```python
from build123d import *

# Parameters (mm, degrees)
SKETCH_1_W           = 150
SKETCH_1_H           = 150
EXTRUDE_2_DEPTH      = 55
CUT_EXTRUDE_1_DEPTH  = 52
SKETCH_3_W           = 20
SKETCH_3_H           = 25.2
CUT_EXTRUDE_2_DEPTH  = 52
SKETCH_4_W           = 31.2
SKETCH_4_H           = 23.663491794
CUT_EXTRUDE_3_DEPTH  = 52
SKETCH_5_W           = 46
SKETCH_5_H           = 120
SKETCH_5_W_2         = 29
CUT_EXTRUDE_4_DEPTH  = 40
SKETCH_6_W           = 3
SKETCH_6_H           = 120
EXTRUDE_4_DEPTH      = 25
SKETCH_7_W           = 3
SKETCH_7_H           = 120
EXTRUDE_5_DEPTH      = 20
CUT_EXTRUDE_6_DEPTH  = 30
FILLET_1_R           = 7
SKETCH_10_W          = 80
SKETCH_10_H          = 50
CUT_EXTRUDE_7_DEPTH  = 30
SKETCH_11_W          = 11.4
SKETCH_11_H          = 20
CUT_EXTRUDE_8_DEPTH  = 30
FILLET_2_R           = 5
FILLET_3_R           = 2
SKETCH_12_W          = 12.6
SKETCH_12_H          = 20
CUT_EXTRUDE_9_DEPTH  = 20
FILLET_4_R           = 2
SKETCH_13_R          = 0.75
CUT_EXTRUDE_10_DEPTH = 5
FILLET_5_R           = 2
FILLET_6_R           = 1
FILLET_8_R           = 0.3


with BuildPart() as part:
    # 草图1 → 凸台-拉伸2 (new body)
    with BuildSketch(Plane.XY):
        with Locations((75, -75)):
            Rectangle(SKETCH_1_W, SKETCH_1_H)
    extrude(amount=EXTRUDE_2_DEPTH)

    # 草图2 → 切除-拉伸1 (cut)
    with BuildSketch(Plane(origin=(0, 0, 0), x_dir=(-1, 0, 0), z_dir=(0, 0, -1))):
        Polygon((-57.4, -53), (-92.6, -53), (-97, -57.4), (-97, -92.6), (-92.6, -97), (-57.4, -97), (-53, -92.6), (-53, -57.4), align=None)
    extrude(amount=-CUT_EXTRUDE_1_DEPTH, mode=Mode.SUBTRACT)

    # 草图3 → 切除-拉伸2 (cut)
    with BuildSketch(Plane(origin=(0, 0, 0), x_dir=(-1, 0, 0), z_dir=(0, 0, -1))):
        with Locations((-43, -75)):
            Rectangle(SKETCH_3_W, SKETCH_3_H)
    extrude(amount=-CUT_EXTRUDE_2_DEPTH, mode=Mode.SUBTRACT)

    # 草图4 → 切除-拉伸3 (cut)
    with BuildSketch(Plane(origin=(0, 0, 0), x_dir=(-1, 0, 0), z_dir=(0, 0, -1))):
        with Locations((-75, -41.168254103)):
            Rectangle(SKETCH_4_W, SKETCH_4_H)
    extrude(amount=-CUT_EXTRUDE_3_DEPTH, mode=Mode.SUBTRACT)

    # 草图5 → 切除-拉伸4 (cut)
    with BuildSketch(Plane(origin=(0, 0, 0), x_dir=(-1, 0, 0), z_dir=(0, 0, -1))):
        with Locations((-127, -75)):
            Rectangle(SKETCH_5_W, SKETCH_5_H)
        with Locations((-164.5, -75)):
            Rectangle(SKETCH_5_W_2, SKETCH_5_H)
    extrude(amount=-CUT_EXTRUDE_4_DEPTH, mode=Mode.SUBTRACT)

    # 草图6 → 凸台-拉伸4 (add)
    with BuildSketch(Plane(origin=(150, 0, 0), x_dir=(0, 0, -1), z_dir=(1, 0, 0))):
        Polygon((-43, -15), (-40, -15), (0, -15), (0, -12), (-43, -12), align=None)
        with Locations((-41.5, -75)):
            Rectangle(SKETCH_6_W, SKETCH_6_H)
        Polygon((0, -135), (-40, -135), (-43, -135), (-43, -138), (0, -138), align=None)
    extrude(amount=EXTRUDE_4_DEPTH)

    # 草图7 → 凸台-拉伸5 (add)
    with BuildSketch(Plane(origin=(0, 0, 40), x_dir=(-1, 0, 0), z_dir=(0, 0, -1))):
        with Locations((-173.5, -75)):
            Rectangle(SKETCH_7_W, SKETCH_7_H)
    extrude(amount=EXTRUDE_5_DEPTH)

    # 草图8 → 切除-拉伸6 (cut)
    with BuildSketch(Plane(origin=(0, 0, 0), x_dir=(-1, 0, 0), z_dir=(0, 0, -1))):
        Polygon((-69, -15), (-104, -15), (-104, -29.336508206), (-90.6, -29.336508206), (-69, -29.336508206), align=None)
    extrude(amount=-CUT_EXTRUDE_6_DEPTH, mode=Mode.SUBTRACT)

    # 圆角1
    fillet_1_edges = [part.edges().sort_by_distance(p)[0] for p in [
        (104, -22.168254103, 30),
        (79.8, -29.336508206, 30),
    ]]
    fillet(fillet_1_edges, radius=FILLET_1_R)

    # 草图10 → 切除-拉伸7 (cut)
    with BuildSketch(Plane(origin=(0, 0, 0), x_dir=(-1, 0, 0), z_dir=(0, 0, -1))):
        with Locations((-52.6, -123.5)):
            Rectangle(SKETCH_10_W, SKETCH_10_H)
    extrude(amount=-CUT_EXTRUDE_7_DEPTH, mode=Mode.SUBTRACT)

    # 草图11 → 切除-拉伸8 (cut)
    with BuildSketch(Plane(origin=(0, 0, 0), x_dir=(-1, 0, 0), z_dir=(0, 0, -1))):
        with Locations((-98.3, -115)):
            Rectangle(SKETCH_11_W, SKETCH_11_H)
    extrude(amount=-CUT_EXTRUDE_8_DEPTH, mode=Mode.SUBTRACT)

    # 圆角2
    fillet_2_edges = [part.edges().sort_by_distance(p)[0] for p in [
        (104, -115, 30),
    ]]
    fillet(fillet_2_edges, radius=FILLET_2_R)

    # 圆角3
    fillet_3_edges = [part.edges().sort_by_distance(p)[0] for p in [
        (90.6, -29.336508206, 15),
        (69, -29.336508206, 18.5),
        (104, -29.336508206, 18.5),
        (104, -125, 17.5),
        (104, -105, 17.5),
        (92.6, -105, 15),
        (92.6, -125, 15),
    ]]
    fillet(fillet_3_edges, radius=FILLET_3_R)

    # 草图12 → 切除-拉伸9 (cut)
    with BuildSketch(Plane(origin=(0, 0, 0), x_dir=(-1, 0, 0), z_dir=(0, 0, -1))):
        with Locations((-6.3, -125)):
            Rectangle(SKETCH_12_W, SKETCH_12_H)
    extrude(amount=-CUT_EXTRUDE_9_DEPTH, mode=Mode.SUBTRACT)

    # 圆角4
    fillet_4_edges = [part.edges().sort_by_distance(p)[0] for p in [
        (12.6, -125, 20),
        (12.6, -135, 10),
        (12.6, -115, 10),
        (0, -125, 20),
        (0, -115, 10),
        (0, -135, 10),
    ]]
    fillet(fillet_4_edges, radius=FILLET_4_R)

    # 草图13 → 切除-拉伸10 (cut)
    with BuildSketch(Plane(origin=(0, 0, 0), x_dir=(-1, 0, 0), z_dir=(0, 0, -1))):
        with Locations((-97, -53)):
            Circle(SKETCH_13_R)
        with Locations(Location((-97, -97, 0), (0, 0, 180))):
            Circle(SKETCH_13_R)
        with Locations((-53, -97)):
            Circle(SKETCH_13_R)
        with Locations(Location((-53, -53, 0), (0, 0, 180))):
            Circle(SKETCH_13_R)
    extrude(amount=-CUT_EXTRUDE_10_DEPTH, mode=Mode.SUBTRACT)

    # 圆角5
    fillet_5_edges = [part.edges().sort_by_distance(p)[0] for p in [
        (175, -13.5, 0),
        (175, -75, 20),
        (175, -15, 10),
        (175, -136.5, 0),
        (175, -135, 10),
    ]]
    fillet(fillet_5_edges, radius=FILLET_5_R)

    # 圆角6
    fillet_6_edges = [part.edges().sort_by_distance(p)[0] for p in [
        (52.6, -148.5, 0),
    ]]
    fillet(fillet_6_edges, radius=FILLET_6_R)

    # 圆角8
    fillet_8_edges = [part.edges().sort_by_distance(p)[0] for p in [
        (12.6, -105.75, 0),
        (0, -143.5, 0),
        (6.3, -135, 0),
        (12.6, -143.25, 0),
        (12.014213562, -135.585786438, 0),
        (0.585786438, -135.585786438, 0),
        (6.3, -115, 0),
        (0.585786438, -114.414213562, 0),
        (12.014213562, -114.414213562, 0),
        (75, 0, 0),
        (150, -144, 0),
        (75, -150, 0),
        (0, -56.5, 0),
        (0, 0, 27.5),
        (150, 0, 27.5),
        (150, -150, 27.5),
        (0, -150, 27.5),
        (150, -6, 0),
    ]]
    fillet(fillet_8_edges, radius=FILLET_8_R)


solid = part.part
```
CAD build for the part. Positions are in the model's coordinates, mm. A direction names the side the tool comes from. Coordinates: 2 decimals unless noted, no trailing zeros. Order: outer loops, then holes, each group sorted by start corner. A loop starts at its lowest first (then second) coordinate and runs counter-clockwise, first axis right, second up. Notation, with made-up numbers: M 37.5,38.25 L 72.5,38.25 A23 ccw 72.5,50.25 Z; hole C -7.5,66 d8. An arc over 180 degrees is marked long. Write each question's results on one line, items separated by ' | '. Start each with the question number.
Q1. Pull direction X, two halves, no side cores. Call faces 1 (the flat face through (43, -87.6, 26)), 2 (the flat face through (0, -76, 27)), 3 (the flat face through (6, -115, 10)): +X half, -X half, draft (parallel to the pull), parting line (faces both ways), or undercut.
Q2. Drill centre lines: probe 1 along Y at (x, z) = (78, 28.5); probe 2 along Y at (x, z) = (48.5, 19.5); probe 3 along Y at (x, z) = (90.5, 51.5). Where is each one in solid material? Low to high. Write a range as from..to.
Q3. Flat gauge pins, fed straight in: P1, Ø9.5, axis at x = 8, y = -121.5, coming from the -Z side; P2, Ø20, axis at x = 161, z = 21, coming from the +Y side; P3, Ø0.8, axis at x = 53, y = -97, coming from the -Z side. Where does each tip first touch, or does it go through?
Q4. Cut at A-A (x = 42). List the corners of the cut face in (y, z), then the cut area to 3 significant figures.
Q5. Cut at B-B (x = 87). List the corners of the cut face in (y, z).
Q6. Which spindle directions (+Z, -Z, +X, -X, +Y, -Y) get a long thin tool onto all of the face, cutting with end or side? Do faces 4 (the flat face through (6, -125, 20)), 5 (the flat face through (55.2, -94.8, 25.6)), 6 (the flat face through (74, -74, 55)). Say none if no direction does.
Found:
1) face 1: undercut | face 2: -X half | face 3: draft
2) probe 1: -150..-148.5, -98.5..-97, -15..0 | probe 2: -150..-148.5, -98.5..-87.6, -62.4..0 | probe 3: -150..-97, -29.34..0
3) P1: z = 20 | P2: y = -12 | P3: z = 5
4) outline: M -150,0.3 A0.3 ccw -149.7,0 L -149.5,0 A1 ccw -148.5,1 L -148.5,30 L -98.5,30 L -98.5,0 L -87.6,0 L -87.6,52 L -62.4,52 L -62.4,0 L -0.3,0 A0.3 ccw 0,0.3 L 0,55 L -150,55 Z | area: 5,440 mm²
5) outline: M -150,0.3 A0.3 ccw -149.7,0 L -149.5,0 A1 ccw -148.5,1 L -148.5,30 L -98.5,30 L -98.5,0 L -97,0 L -97,52 L -29.34,52 L -29.34,37 A7 ccw -22.34,30 L -15,30 L -15,0 L -0.3,0 A0.3 ccw 0,0.3 L 0,55 L -150,55 Z
6) face 4: -Z, -X | face 5: -Z | face 6: +Z, +X, -X, +Y, -Y
